Part model, mm, in its own coordinate system. A direction names the side the tool comes from. Round coordinates to 2 decimals unless told otherwise and drop trailing zeros. Order: outer loops, then holes, each group sorted by start corner. A loop starts at its lowest first (then second) coordinate and runs counter-clockwise, first axis right, second up. Notation, with made-up numbers: M 46.25,85.5 L 101.25,85.5 A13 ccw 101.25,108.5 Z; hole C 36.25,-13.75 d6. An arc over 180 degrees is marked long. One line per question, with ' | ' between items.
from build123d import *

# Parameters (mm, degrees)
SKETCH_1_R          = 3
EXTRUDE_1_DEPTH     = 6
SKETCH_2_R          = 65
CUT_EXTRUDE_1_DEPTH = 3
CUT_EXTRUDE_1_DRAFT = -60
SKETCH_3_OUTSIDE_W  = 166.354
SKETCH_3_OUTSIDE_H  = 166.354
SKETCH_3_OUTSIDE_R  = 62.5
CUT_EXTRUDE_2_DEPTH = 3
CUT_EXTRUDE_2_DRAFT = -60
CUT_EXTRUDE1_DEPTH  = 86.064681421


with BuildPart() as part:
    # Эскиз1 → Бобышка-Вытянуть1 (new body)
    with BuildSketch(Plane(origin=(0, 0, 0), x_dir=(1, 0, 0), z_dir=(0, 1, 0))):
        with BuildLine():
            Line((-51.514718626, -60), (-37.971101151, -46.456382526))
            ThreePointArc((-37.971101151, -46.456382526), (0, -60), (37.971101151, -46.456382526))
            Line((37.971101151, -46.456382526), (51.514718626, -60))
            Line((51.514718626, -60), (60, -60))
            Line((60, -60), (60, -51.514718626))
            Line((60, -51.514718626), (46.456382526, -37.971101151))
            ThreePointArc((46.456382526, -37.971101151), (60, 0), (46.456382526, 37.971101151))
            Line((46.456382526, 37.971101151), (60, 51.514718626))
            Line((60, 51.514718626), (60, 60))
            Line((60, 60), (51.514718626, 60))
            Line((51.514718626, 60), (37.971101151, 46.456382526))
            ThreePointArc((37.971101151, 46.456382526), (0, 60), (-37.971101151, 46.456382526))
            Line((-37.971101151, 46.456382526), (-51.514718626, 60))
            Line((-51.514718626, 60), (-60, 60))
            Line((-60, 60), (-60, 51.514718626))
            Line((-60, 51.514718626), (-46.456382526, 37.971101151))
            ThreePointArc((-46.456382526, 37.971101151), (-60, 0), (-46.456382526, -37.971101151))
            Line((-46.456382526, -37.971101151), (-60, -51.514718626))
            Line((-60, -51.514718626), (-60, -60))
            Line((-60, -60), (-51.514718626, -60))
        make_face()
        with Locations(Location((-52.5, -52.5, 0), (0, 0, 270))):
            Circle(SKETCH_1_R, mode=Mode.SUBTRACT)
        with Locations(Location((-52.5, 52.5, 0), (0, 0, 270))):
            Circle(SKETCH_1_R, mode=Mode.SUBTRACT)
        with Locations(Location((52.5, 52.5, 0), (0, 0, 270))):
            Circle(SKETCH_1_R, mode=Mode.SUBTRACT)
        with Locations(Location((52.5, -52.5, 0), (0, 0, 270))):
            Circle(SKETCH_1_R, mode=Mode.SUBTRACT)
        with BuildLine():
            Line((2.73923518, 6.981875867), (6.459180807, 10.701821494))
            ThreePointArc((6.459180807, 10.701821494), (0, 12.5), (-6.459180807, 10.701821494))
            Line((-6.459180807, 10.701821494), (-2.73923518, 6.981875867))
            ThreePointArc((-2.73923518, 6.981875867), (0, 7.5), (2.73923518, 6.981875867))
        make_face(mode=Mode.SUBTRACT)
    extrude(amount=EXTRUDE_1_DEPTH)


with BuildPart() as cut_extrude_1_tool:
    # Эскиз2 → Вырез-Вытянуть1 (with draft: the straight prism first)
    with BuildSketch(Plane.XZ):
        Circle(SKETCH_2_R)
    extrude(amount=-CUT_EXTRUDE_1_DEPTH)
    # Вырез-Вытянуть1: the draft: its side faces are tilted about the plane it starts from
    cut_extrude_1_sides = [cut_extrude_1_tool.faces().sort_by_distance(p)[0] for p in [
        (-65, 1.5, 0),
    ]]
    draft(cut_extrude_1_sides, Plane.XZ, CUT_EXTRUDE_1_DRAFT)


with BuildPart() as part_1:
    add(part.part)

    # Вырез-Вытянуть1: cut by cut_extrude_1_tool
    add(cut_extrude_1_tool.part, mode=Mode.SUBTRACT)


with BuildPart() as cut_extrude_2_tool:
    # Эскиз3 outside → Вырез-Вытянуть2 (with draft: the straight prism first)
    with BuildSketch(Plane(origin=(0, 6, 0), x_dir=(1, 0, 0), z_dir=(0, 1, 0))):
        Rectangle(SKETCH_3_OUTSIDE_W, SKETCH_3_OUTSIDE_H)
        Circle(SKETCH_3_OUTSIDE_R, mode=Mode.SUBTRACT)
    extrude(amount=-CUT_EXTRUDE_2_DEPTH)
    # Вырез-Вытянуть2: the draft: its side faces are tilted about the plane it starts from
    cut_extrude_2_sides = [cut_extrude_2_tool.faces().sort_by_distance(p)[0] for p in [
        (0, 4.5, 83.177),
        (83.177, 4.5, 0),
        (0, 4.5, -83.177),
        (-83.177, 4.5, 0),
        (-62.5, 4.5, 0),
    ]]
    draft(cut_extrude_2_sides, Plane(origin=(0, 6, 0), x_dir=(1, 0, 0), z_dir=(0, 1, 0)), CUT_EXTRUDE_2_DRAFT)


with BuildPart() as part_2:
    add(part_1.part)

    # Вырез-Вытянуть2: cut by cut_extrude_2_tool
    add(cut_extrude_2_tool.part, mode=Mode.SUBTRACT)

    # Sketch1 → Cut-Extrude1 (cut, through all)
    with BuildSketch(Plane(origin=(0, 6, 0), x_dir=(1, 0, 0), z_dir=(0, 1, 0))):
        Polygon((19.45563956, 53.914075196), (5.07363956, 45.610623625), (19.45563956, 37.307172053), (33.83763956, 45.610623625), align=None)
        Polygon((2.53563956, 41.214678675), (2.53563956, 24.607775532), (16.91763956, 16.30432396), (16.91763956, 32.911227103), align=None)
        Polygon((21.99363956, 16.30432396), (36.37563956, 24.607775532), (36.37563956, 41.214678675), (21.99363956, 32.911227103), align=None)
        Polygon((-19.46036044, 53.914075196), (-33.84236044, 45.610623625), (-19.46036044, 37.307172053), (-5.07836044, 45.610623625), align=None)
        Polygon((-36.38036044, 41.214678675), (-36.38036044, 24.607775532), (-21.99836044, 16.30432396), (-21.99836044, 32.911227103), align=None)
        Polygon((-16.92236044, 16.30432396), (-2.54036044, 24.607775532), (-2.54036044, 41.214678675), (-16.92236044, 32.911227103), align=None)
        Polygon((38.91363956, 20.211830582), (24.53163956, 11.908379011), (38.91363956, 3.604927439), (53.29563956, 11.908379011), align=None)
        Polygon((21.99363956, 7.512434061), (21.99363956, -9.094469082), (36.37563956, -17.397920653), (36.37563956, -0.79101751), align=None)
        Polygon((41.45163956, -17.397920653), (55.83363956, -9.094469082), (55.83363956, 7.512434061), (41.45163956, -0.79101751), align=None)
        Polygon((-2.54036044, -42.796713695), (-16.92236044, -51.100165267), (-16.92236044, -34.493262124), (-2.54036044, -26.189810552), align=None)
        Polygon((19.45563956, -13.490414031), (5.07363956, -21.793865603), (19.45563956, -30.097317174), (33.83763956, -21.793865603), align=None)
        Polygon((2.53563956, -26.189810552), (2.53563956, -42.796713695), (16.91763956, -51.100165267), (16.91763956, -34.493262124), align=None)
        Polygon((21.99363956, -51.100165267), (36.37563956, -42.796713695), (36.37563956, -26.189810552), (21.99363956, -34.493262124), align=None)
        Polygon((-19.46036044, -13.490414031), (-33.84236044, -21.793865603), (-19.46036044, -30.097317174), (-5.07836044, -21.793865603), align=None)
        Polygon((-36.38036044, -26.189810552), (-36.38036044, -42.796713695), (-21.99836044, -51.100165267), (-21.99836044, -34.493262124), align=None)
        Polygon((-21.99836044, -9.094469082), (-36.38036044, -17.397920653), (-36.38036044, -0.79101751), (-21.99836044, 7.512434061), align=None)
        Polygon((-0.00236044, 20.211830582), (-14.38436044, 11.908379011), (-0.00236044, 3.604927439), (14.37963956, 11.908379011), align=None)
        Polygon((-16.92236044, 7.512434061), (-16.92236044, -9.094469082), (-2.54036044, -17.397920653), (-2.54036044, -0.79101751), align=None)
        Polygon((2.53563956, -17.397920653), (16.91763956, -9.094469082), (16.91763956, 7.512434061), (2.53563956, -0.79101751), align=None)
        Polygon((-38.91836044, 20.211830582), (-53.30036044, 11.908379011), (-38.91836044, 3.604927439), (-24.53636044, 11.908379011), align=None)
        Polygon((-55.83836044, 7.512434061), (-55.83836044, -9.094469082), (-41.45636044, -17.397920653), (-41.45636044, -0.79101751), align=None)
    extrude(amount=-CUT_EXTRUDE1_DEPTH, mode=Mode.SUBTRACT)


solid = part_2.part
1) Two-plate mould, pull along X, no slides. Class faces 5 (the face through (53, 3, -56)), 6 (the face through (-12.17, 4.52, 17.7)), 7 (the face through (59.997, 4.422, 0.576)): released by +X, released by -X, zero draft, split by the parting line, or undercut.
The answers:
face 5: zero draft | face 6: undercut | face 7: released by +X
2) Probe line 1 (Z direction, x = 52.5, y = 4.25); line 2 (X direction, y = 1.8, z = -52.5); line 3 (Z direction, x = 19, y = 3.5). List the from-to ranges inside material, lowest first. Write a range as [from, to].
The answers:
line 1: z = [-29.05, -12.37], [-11.45, -5.59], [11.02, 29.05] | line 2: x = [-60, -55.5], [-49.5, -44.01], [44.01, 49.5], [55.5, 60] | line 3: z = [-56.91, -53.65], [-37.57, 13.75], [29.83, 56.91]
3) Which spindle directions (+Z, -Z, +X, -X, +Y, -Y) get a long thin tool onto all of the face, cutting with end or side? Do faces 1 (the face through (-53.323, 2.291, -44.838)), 2 (the face through (-26.551, 4.521, 17.584)), 3 (the face through (-44.838, 2.291, 53.323)), 4 (the face through (-60, 1, 56)). Say none if no direction does.
The answers:
face 1: -X, +Y, -Y | face 2: +Y, -Y | face 3: +Z, +Y, -Y | face 4: +Z, -Z, -X, +Y, -Y
4) Saw through at B-B (x = -27). Give the number of separate pieces and of enclosed holes in the cut face, plus the area to 3 significant figures.
The answers:
separate pieces: 7 | enclosed holes: 0 | area: 116 mm²
5) Drop flat-ended pins along their axis: pin 1 (0.9 mm diameter, centred on y = 4.5, z = -21.5, fed in from -X); pin 2 (1.5 mm diameter, centred on y = 4, z = 45, fed in from -X); pin 3 (1.5 mm diameter, centred on y = 5, z = 0.5, fed in from +X); pin 4 (1.5 mm diameter, centred on x = -9, y = 4, fed in from -Z). Give the stop position or say it passes through.
The answers:
pin 1: stops at x = -56.19 | pin 2: stops at x = -50.12 | pin 3: stops at x = 60 | pin 4: stops at z = -59.43
6) Saw through at A-A (y = 1.25). List the corners of the cut face in (x, z), plus the area to 3 significant figures.
The answers:
outline: M -60,-60 L -51.51,-60 L -39.99,-48.47 A62.83 cw -48.47,-39.99 L -60,-51.51 Z; M -60,51.51 L -48.47,39.99 A62.83 cw -39.99,48.47 L -51.51,60 L -60,60 Z; M 39.99,-48.47 L 51.51,-60 L 60,-60 L 60,-51.51 L 48.47,-39.99 A62.83 cw Z; M 39.99,48.47 A62.83 cw 48.47,39.99 L 60,51.51 L 60,60 L 51.51,60 Z; hole C -52.5,-52.5 d6; hole C -52.5,52.5 d6; hole C 52.5,-52.5 d6; hole C 52.5,52.5 d6 | area: 804 mm²
